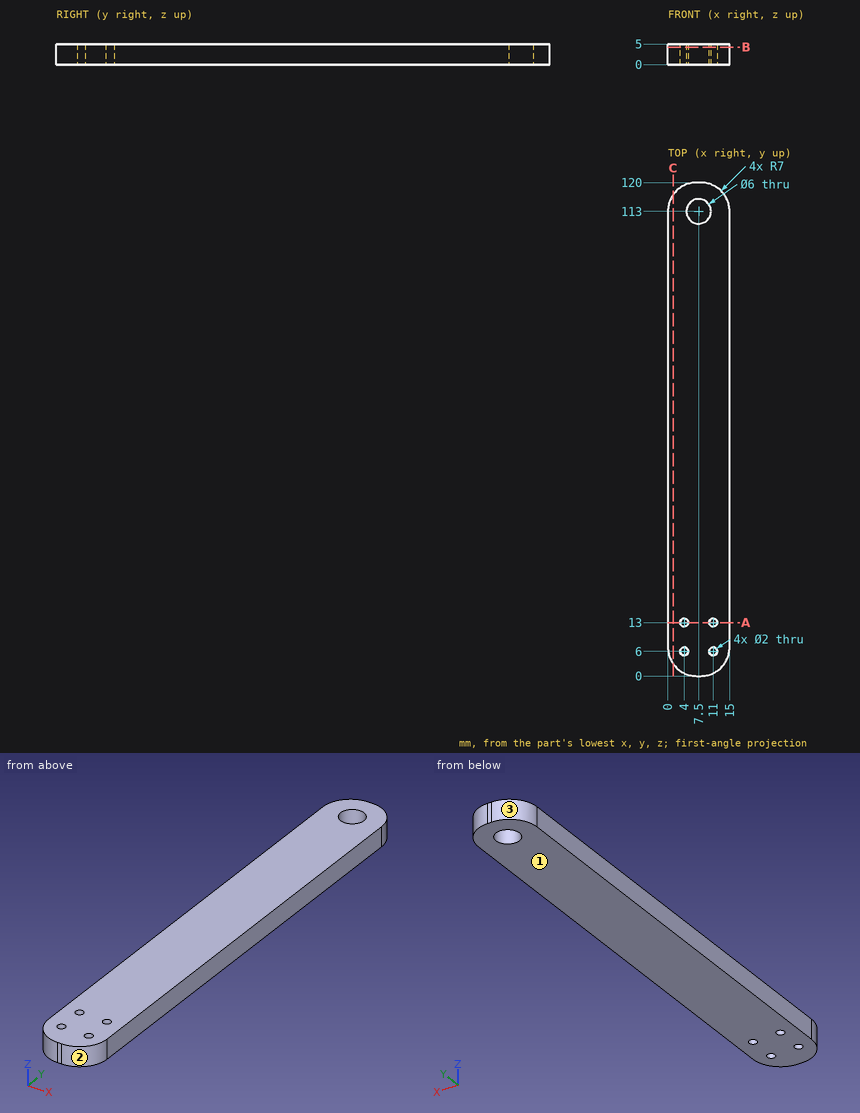
Part print with two shaded views. Sizes in mm from the minimum x, y, z corner. Coordinates: 2 decimals unless noted, no trailing zeros. Write each loop counter-clockwise with the first axis right and the second up, starting at its lowest first coordinate (ties: lowest second). Pieces come first, ordered by that corner, then holes. Notation, with made-up numbers: (46.25, 36) - (96.25, 36) arc R13 cw to (96.25, 49) - close; hole circle Ø5 at (-35.5, -6). An arc over 180 degrees is marked (long way). One line per item, written item: value. Start each with the question number.
1. Slice it at C-C (x = 1.25). Write the cut outline in (y, z).
2. Slice it at A-A (y = 13). Write the cut outline in (x, z), plus the area to 3 significant figures.
3. Probe line 1 (X direction, y = 13, z = 3.1); line 2 (Y direction, x = 4, z = 1.85); line 3 (Y direction, x = 11.25, z = 3.4). List the from-to ranges inside material, lowest first. Write a range as from..to.
4. Flat gauge pins, fed straight in: pin 1 (1.5 mm diameter, centred on x = 5, z = 4, fed in from -Y); pin 2 (5.5 mm diameter, centred on x = 7.5, y = 113, fed in from -Z). Where does each tip first touch, or does it go through?
5. Slice it at B-B (z = 4.25). Write the cut outline in (x, y), plus the area to 3 significant figures.
6. Mould opens along Y. For the marked faces 1, 2 and 3 say: released by +Y, released by -Y, zero draft, split by the parting line, or undercut.
Answers below:
1. outline: (3.01, 0) - (116.99, 0) - (116.99, 5) - (3.01, 5) - close
2. outline: (0, 0) - (3, 0) - (3, 5) - (0, 5) - close; (5, 0) - (10, 0) - (10, 5) - (5, 5) - close; (12, 0) - (15, 0) - (15, 5) - (12, 5) - close
2. area: 55.0 mm^2
3. line 1: x = 0..3, 5..10, 12..15
3. line 2: y = 0.68..5, 7..12, 14..119.32
3. line 3: y = 0.8..5.03, 6.97..12.03, 13.97..119.2
4. pin 1: stops at y = 0.11
4. pin 2: passes through
5. outline: (0, 7) arc R7 ccw to (7, 0) - (8, 0) arc R7 ccw to (15, 7) - (15, 113) arc R7 ccw to (8, 120) - (7, 120) arc R7 ccw to (0, 113) - close; hole circle Ø2 at (4, 6); hole circle Ø2 at (4, 13); hole circle Ø6 at (7.5, 113); hole circle Ø2 at (11, 6); hole circle Ø2 at (11, 13)
5. area: 1,720 mm^2
6. face 1: zero draft
6. face 2: released by -Y
6. face 3: released by +Y
